```python
from build123d import *

# Parameters (mm, degrees)
F0_W     = 26
F0_H     = 26
F1_DEPTH = 1.5
F2_W     = 5
F2_H     = 26
F3_DEPTH = 3
F4_R     = 3
F5_DEPTH = 25
F6_DEPTH = 24
F7_W     = 50
F7_H     = 1.5
F8_DEPTH = 44


with BuildPart() as f1:
    # F0 (on Front) → F1 (new body)
    with BuildSketch(Plane.XZ):
        Rectangle(F0_W, F0_H)
    extrude(amount=-F1_DEPTH)

    # F2 (on face) → F3 (join)
    with BuildSketch(Plane(origin=(0, 1.5, 0), x_dir=(-1, 0, 0), z_dir=(0, 1, 0))):
        with Locations((4.25, 0)):
            Rectangle(F2_W, F2_H)
    extrude(amount=F3_DEPTH)

    # F4 (on face) → F5 (cut)
    with BuildSketch(Plane.XZ):
        with Locations((5.25, 5.75)):
            Circle(F4_R)
    extrude(amount=-F5_DEPTH, mode=Mode.SUBTRACT)

    # F6 (add): a face of the model
    f6_faces = [f1.faces().sort_by_distance(p)[0] for p in [
        (13, 0.75, 0),
    ]]
    extrude(f6_faces, amount=F6_DEPTH)

    # F7 (on face) → F8 (join)
    with BuildSketch(Plane(origin=(0, 0, -13), x_dir=(1, 0, 0), z_dir=(0, 0, -1))):
        with Locations((12, -0.75)):
            Rectangle(F7_W, F7_H)
    extrude(amount=F8_DEPTH)


solid = f1.part
```
Work out the finished part from the listing and answer in its coordinate system (mm). A direction names the side the tool comes from. Round coordinates to 2 decimals unless told otherwise and drop trailing zeros. Loops run counter-clockwise (first coordinate to the right, second up) from the corner with the lowest first, then second, coordinate; pieces in that order, holes last. Notation, with made-up numbers: M 16,69 L 29,69 A15 cw 29,75 Z; hole C 10,-24 d5. An arc over 180 degrees is marked long. Use CSV: the item, a comma, the result in double quotes.
Q1. Section B-B, the plane z = 5.75 is taken. Determine the outline of the cut face in (x, y).
Determined:
outline,"M -13,0 L 2.25,0 L 2.25,1.5 L -1.75,1.5 L -1.75,4.5 L -6.75,4.5 L -6.75,1.5 L -13,1.5 Z; M 8.25,0 L 37,0 L 37,1.5 L 8.25,1.5 Z"
Q2. Section D-D, the plane y = 3.1 is taken. Determine the outline of the cut face in (x, z).
Determined:
outline,"M -6.75,-13 L -1.75,-13 L -1.75,13 L -6.75,13 Z"
Q3. Each of these flat-tipped pins is pushed along its axis until it touches: pin 1 (6 mm diameter, centred on x = 30, z = -46, fed in from +Y); pin 2 (2.5 mm diameter, centred on y = 3.5, z = -3.5, fed in from -X); pin 3 (0.9 mm diameter, centred on x = -4, y = 3.5, fed in from -Z); pin 4 (1.5 mm diameter, centred on y = 2.5, z = -14, fed in from -X). Where does it stop, or does it pass through?
Determined:
pin 1,"y = 1.5"
pin 2,"x = -6.75"
pin 3,"z = -13"
pin 4,"through"
Q4. Section C-C, the plane z = -3 is taken. Determine the outline of the cut face in (x, y), then the cut area to 3 significant figures.
Determined:
outline,"M -13,0 L 37,0 L 37,1.5 L -1.75,1.5 L -1.75,4.5 L -6.75,4.5 L -6.75,1.5 L -13,1.5 Z"
area,"90.0 mm2"
Q5. Section A-A, the plane x = 5.25 is taken. Determine the outline of the cut face in (y, z), then the cut area to 3 significant figures.
Determined:
outline,"M 0,-57 L 1.5,-57 L 1.5,2.75 L 0,2.75 Z; M 0,8.75 L 1.5,8.75 L 1.5,13 L 0,13 Z"
area,"96.0 mm2"
Q6. A tool of negligible diameter and unlimited length cuts with its end or side. For faces 1 (the flat face through (-6.75, 3, 0)), 2 (the flat face through (-4, 3, -13)), 3 (the flat face through (-1.75, 3, 0)), from which of +Z, -Z, +X, -X, +Y, -Y can it reach the whole face along a straight path? Write none if from no direction.
Determined:
face 1,"+Z, -Z, -X, +Y"
face 2,"-Z, +X, -X, +Y"
face 3,"+Z, -Z, +X, +Y"
Q7. The mould has two halves that part along X. Classify faces 4 (the cylindrical face through (6.634, 0.74, 3.088)), 5 (the flat face through (12, 1, -57)), 6 (the flat face through (-13, 1, -22)): pulls with the +X half, pulls with the -X half, needs draft (parallel to the pull), parting line crosses it, or undercut.
Determined:
face 4,"undercut"
face 5,"needs draft"
face 6,"pulls with the -X half"
Q8. Consider L1, parallel to Z at x = 5.25, y = 0.9; L2, parallel to Y at x = 25.5, z = -23; L3, parallel to X at y = 1.65, z = -1. Determine where each line is inside the solid, lowest interval first.
Determined:
L1,"-57 to 2.75, 8.75 to 13"
L2,"0 to 1.5"
L3,"-6.75 to -1.75"
